Work out the finished part from the listing and answer in its coordinate system (mm). Face numbers are marked on the shaded views. A direction names the side the tool comes from. Round coordinates to 2 decimals unless told otherwise and drop trailing zeros. Write each loop counter-clockwise with the first axis right and the second up, starting at its lowest first coordinate (ties: lowest second). Pieces come first, ordered by that corner, then holes. Notation, with made-up numbers: (51.25, 50.5) - (66.25, 50.5) arc R22 ccw to (66.25, 81.5) - close; hole circle Ø9 at (-20, 63.25). An arc over 180 degrees is marked (long way). Answer as a JSON object with one key per item and string values.
Autodesk Inventor part; units mm, degrees
ref_plane "YZ Plane" through (0, 0, 0) normal (1, 0, 0) x (0, 1, 0)
ref_plane "XZ Plane" through (0, 0, 0) normal (0, 1, 0) x (-1, 0, 0)
ref_plane "XY Plane" through (0, 0, 0) normal (0, 0, 1) x (1, 0, 0)
sketch "Skizze1" plane through (0, 0, 0) normal (0, 0, 1) x (1, 0, 0)
  line L0 (0, 0) -> (100, 0)
  line L1 (100, 0) -> (100, 4)
  line L2 (100, 4) -> (0, 4)
  line L3 (0, 4) -> (0, 0)
  dimension "d0" = 100
  dimension "d1" = 4
extrude "Extrusion1" add sketch "Skizze1" along normal blind 20
sketch "Skizze2" plane through (0, 0, 0) normal (0, 0, -1) x (-1, 0, 0)
  line L0 (0, 4) -> (0, 0)
  line L1 (-100, 4) -> (0, 4)
  line L2 (0, 4) -> (2.5, 4) construction
  line L3 (1.7678, 5.7678) -> (1.7678, 5.75)
  arc A0 (2.8969, 2.663) -> (0.0178, 4) centre (1.7678, 4) ccw
  line L4 (0, 0) -> (3.0052, 2.7626)
  line L5 (0, 4) -> (0.0179, 4.0179)
  line L6 (1.7499, 5.7499) -> (1.7678, 5.7678)
  circle A1 centre (1.7678, 4) radius 0.75
  dimension "d4" = 2.5
  dimension "d6" = 3.5
  dimension "d9" = 1.5
extrude "Extrusion2" add sketch "Skizze2" against normal blind 20 contours L5 A0 L4 L0 | A1
sketch "Skizze3" plane through (0, 0, 0) normal (0, 0, -1) x (-1, 0, 0)
  point P0 (0, 0)
extrude "Extrusion3" cut sketch "Skizze2" against normal blind 20 contours A1
sketch "Skizze4" plane through (100, 0, 0) normal (0, -1, 0) x (1, 0, 0)
  line L0 (0, 20) -> (-100, 20)
  line L1 (0, 0) -> (-100, 0)
  line L2 (0, 20) -> (-2, 20)
  line L3 (-2, 20) -> (-2, 0)
  line L4 (-2, 0) -> (0, 0)
  line L5 (0, 0) -> (0, 20)
  dimension "d12" = 2
extrude "Extrusion4" add sketch "Skizze4" along normal blind 5
sketch "Skizze6" plane through (0, 0, 0) normal (0, -1, 0) x (1, 0, 0)
  line L0 (0, 0) -> (0, 20)
  line L1 (0, 20) -> (0, 15)
  line L2 (0, 15) -> (0, 10)
  line L3 (0, 10) -> (0, 5)
  line L4 (0, 5) -> (0, 0)
  line L5 (-3.5178, 0) -> (-0.0179, 0)
  line L6 (0, 0) -> (-3.5178, 0)
  line L7 (-3.5178, 0) -> (-3.5178, 5)
  line L8 (-3.5178, 0) -> (-3.5178, 20)
  line L9 (0, 5) -> (-3.5178, 5)
  line L10 (0, 15) -> (-3.5178, 15)
  line L11 (-3.5178, 15) -> (-3.5178, 10)
  line L12 (0, 10) -> (-3.5178, 10)
  point P0 (-3.0052, 0)
  dimension "d22" = 5
  dimension "d23" = 5
  dimension "d24" = 5
extrude "Extrusion5" cut sketch "Skizze6" against normal blind 50 contours L6 L5 L7 L9 L0 | L12 L8 L10 L0
properties part number "Hebel_Klemme_oben"
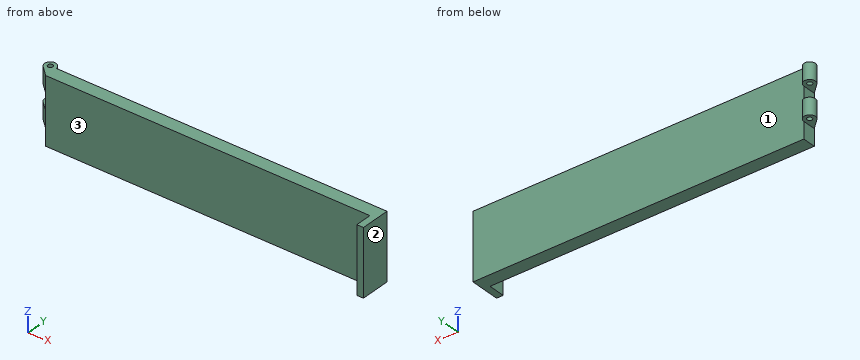
Item 1: Each of these flat-tipped pins is pushed along its axis until it touches: P1, Ø2.5, axis at y = -1.5, z = 13.5, coming from the -X side; P2, Ø10, axis at x = 18.5, z = 16.5, coming from the -Y side; P3, Ø2, axis at x = -1.77, y = 4, coming from the -Z side. Where does it stop, or does it pass through?
Results found:
{"P1": "x = 98", "P2": "y = 0", "P3": "z = 5"}
Item 2: A cutting plane is placed at D-D (x = 33). Write down the section's boundary in (y, z), and give its area (3 significant figures).
Results found:
{"outline": "(0, 0) - (4, 0) - (4, 20) - (0, 20) - close", "area": "80.0 mm²"}
Item 3: A cutting plane is placed at B-B (y = 1.5). Write down the section's boundary in (x, z), and give its area (3 significant figures).
Results found:
{"outline": "(-1.63, 5) - (0, 5) - (0, 0) - (100, 0) - (100, 20) - (-1.63, 20) - (-1.63, 15) - (0, 15) - (0, 10) - (-1.63, 10) - close", "area": "2,020 mm²"}
Item 4: A cutting plane is placed at A-A (z = 13.75). Write down the section's boundary in (x, y).
Results found:
{"outline": "(0, 0) - (98, 0) - (98, -5) - (100, -5) - (100, 4) - (0, 4) - close"}
Item 5: For the marked faces 1, 2 and 3, determine the directions among +Z, -Z, +X, -X, +Y, -Y from which every point of the face is accessible in a straight line to the end or side of a thin tool.
Results found:
{"face 1": "+Z, -Z, +X, +Y", "face 2": "+Z, -Z, +X, +Y, -Y", "face 3": "+Z, -Z, -X, -Y"}
Item 6: Consider line 1 along Y through (x, z) = (12, 5.75); line 2 along X through (y, z) = (-2, 6); line 3 along X through (y, z) = (3, 13.75). Determine where each line is inside the solid, lowest interval first.
Results found:
{"line 1": "0 to 4", "line 2": "98 to 100", "line 3": "0 to 100"}
